```python
from build123d import *

# Parameters (mm, degrees)
SKETCH1_W           = 304.8
SKETCH1_H           = 50.8
BOSS_EXTRUDE1_DEPTH = 6.35
SKETCH2_W           = 41.275
SKETCH2_H           = 22.225
CUT_EXTRUDE1_DEPTH  = 265.034300402
SKETCH5_W           = 25.4
SKETCH5_H           = 6.35
BOSS_EXTRUDE2_DEPTH = 6.35
LPATTERN1_COUNT     = 6
LPATTERN1_PITCH     = 50.8
SKETCH6_W           = 6.35
SKETCH6_H           = 12.7
BOSS_EXTRUDE3_DEPTH = 6.35
LPATTERN2_COUNT     = 2
LPATTERN2_PITCH     = 38.1
CUT_EXTRUDE2_DEPTH  = 272.024068837
CUT_EXTRUDE3_DEPTH  = 272.024068837
SKETCH9_R           = 2.0955
CUT_EXTRUDE4_DEPTH  = 272.024068837


with BuildPart() as part:
    # Sketch1 → Boss-Extrude1 (new body)
    with BuildSketch(Plane.XY):
        with Locations((-110.333, 0)):
            Rectangle(SKETCH1_W, SKETCH1_H)
    extrude(amount=BOSS_EXTRUDE1_DEPTH)

    # Sketch2 → Cut-Extrude1 (cut, through all)
    with BuildSketch(Plane.XY.offset(6.35)):
        Rectangle(SKETCH2_W, SKETCH2_H)
    extrude(amount=-CUT_EXTRUDE1_DEPTH, mode=Mode.SUBTRACT)

    # Sketch5 → Boss-Extrude2 (add)
    with BuildSketch(Plane.XZ.offset(25.4)):
        with Locations((3.967, 3.175)):
            Rectangle(SKETCH5_W, SKETCH5_H)
    boss_extrude2 = extrude(amount=BOSS_EXTRUDE2_DEPTH)

    # LPattern1: Boss-Extrude2 ×6
    with Locations(*[(-i * LPATTERN1_PITCH, 0, 0) for i in range(1, LPATTERN1_COUNT)]):
        add(boss_extrude2)

    # Sketch6 → Boss-Extrude3 (add)
    with BuildSketch(Plane.ZY.offset(262.733)):
        with Locations((3.175, 19.05)):
            Rectangle(SKETCH6_W, SKETCH6_H)
    boss_extrude3 = extrude(amount=BOSS_EXTRUDE3_DEPTH)

    # LPattern2: Boss-Extrude3 ×2
    with Locations(*[(0, -i * LPATTERN2_PITCH, 0) for i in range(1, LPATTERN2_COUNT)]):
        add(boss_extrude3)

    # Sketch7 → Cut-Extrude2 (cut, through all)
    with BuildSketch(Plane.XY.offset(6.35)):
        Polygon((-262.733, 2.1336), (-262.733, -2.1336), (-253.97, -2.1336), (-253.97, -4.445), (-250.795, -4.445), (-250.795, -2.1336), (-247.493, -2.1336), (-247.493, 2.1336), (-250.795, 2.1336), (-250.795, 4.445), (-253.97, 4.445), (-253.97, 2.1336), align=None)
    extrude(amount=-CUT_EXTRUDE2_DEPTH, mode=Mode.SUBTRACT)

    # Sketch8 → Cut-Extrude3 (cut, through all)
    with BuildSketch(Plane.XY.offset(6.35)):
        Polygon((-226.7666, -25.4), (-222.4994, -25.4), (-222.4994, -16.637), (-220.188, -16.637), (-220.188, -13.462), (-222.4994, -13.462), (-222.4994, -10.16), (-226.7666, -10.16), (-226.7666, -13.462), (-229.078, -13.462), (-229.078, -16.637), (-226.7666, -16.637), align=None)
        Polygon((-125.1666, -25.4), (-120.8994, -25.4), (-120.8994, -16.637), (-118.588, -16.637), (-118.588, -13.462), (-120.8994, -13.462), (-120.8994, -10.16), (-125.1666, -10.16), (-125.1666, -13.462), (-127.478, -13.462), (-127.478, -16.637), (-125.1666, -16.637), align=None)
        Polygon((27.2334, -25.4), (31.5006, -25.4), (31.5006, -16.637), (33.812, -16.637), (33.812, -13.462), (31.5006, -13.462), (31.5006, -10.16), (27.2334, -10.16), (27.2334, -13.462), (24.922, -13.462), (24.922, -16.637), (27.2334, -16.637), align=None)
    extrude(amount=-CUT_EXTRUDE3_DEPTH, mode=Mode.SUBTRACT)

    # Sketch9 → Cut-Extrude4 (cut, through all)
    with BuildSketch(Plane(origin=(0, 0, 0), x_dir=(-1, 0, 0), z_dir=(0, 0, -1))):
        with Locations((46.904309807, -28.575)):
            Circle(SKETCH9_R)
        with Locations((199.304309807, -28.575)):
            Circle(SKETCH9_R)
    extrude(amount=-CUT_EXTRUDE4_DEPTH, mode=Mode.SUBTRACT)


solid = part.part
```
CAD build for the part. Positions are in the model's coordinates, mm. A direction names the side the tool comes from. Round coordinates to 2 decimals unless told otherwise and drop trailing zeros. Order: outer loops, then holes, each group sorted by start corner. A loop starts at its lowest first (then second) coordinate and runs counter-clockwise, first axis right, second up. Notation, with made-up numbers: (33, -36.75) - (53, -36.75) arc R26 ccw to (53, -15.75) - close; hole circle Ø9 at (62, 3.5). An arc over 180 degrees is marked (long way). Answer as CSV lines item,"result". Start each with the question number.
1. Saw through at A-A, the plane y = -20. Write the cut outline in (x, z).
2. Pin check, flat tips, straight feed: pin 1 (1.2 mm diameter, centred on x = 32.5, z = 4.5, fed in from -Y); pin 2 (1.8 mm diameter, centred on y = 3.5, z = 2, fed in from -X). Stop position of each tip, or through.
3. Drill centre lines: L1, parallel to X at y = -26, z = 4.75; L2, parallel to X at y = -11, z = 6; L3, parallel to X at y = -4, z = 1 (1 decimal). Where is each one in solid material? Low to high. Write a range as [from, to].
4. Pull direction X, two halves, no side cores. Call faces 6 (the face through (-161.133, -29, 3)), 7 (the face through (16.667, -29, 3)), 8 (the face through (37, -25.4, 3)): +X half, -X half, draft (parallel to the pull), parting line (faces both ways), or undercut.
5. Saw through at C-C, the plane y = -7. Write the cut outline in (x, z).
6. Saw through at B-B, the plane x = -6. Write the cut outline in (y, z), and give its area (3 significant figures).
7. Tool access for faces 1 (the face through (-262.733, 7, 3)), 2 (the face through (-237.333, -29, 3)), 3 (the face through (-20.638, 0, 3)), 4 (the face through (-266, -25.4, 3)), 5 (the face through (-111, -4, 6.35)): list every direction of +Z, -Z, +X, -X, +Y, -Y with a clear straight run to the whole face (end or side of a thin tool).
8. Saw through at D-D, the plane z = 2.75. Count the separate pieces of the cut face and the enclosed holes in it, and give its area (3 significant figures).
Model answer:
1,outline,"(-269.08, 0) - (-226.77, 0) - (-226.77, 6.35) - (-269.08, 6.35) - close; (-222.5, 0) - (-125.17, 0) - (-125.17, 6.35) - (-222.5, 6.35) - close; (-120.9, 0) - (27.23, 0) - (27.23, 6.35) - (-120.9, 6.35) - close; (31.5, 0) - (42.07, 0) - (42.07, 6.35) - (31.5, 6.35) - close"
2,pin 1,"stops at y = -25.4"
2,pin 2,"stops at x = -262.73"
3,L1,"x = [-262.73, -237.33], [-211.93, -186.53], [-161.13, -135.73], [-110.33, -84.93], [-59.53, -34.13], [-8.73, 16.67]"
3,L2,"x = [-262.73, -226.77], [-222.5, -125.17], [-120.9, -20.64], [20.64, 27.23], [31.5, 42.07]"
3,L3,"x = [-262.7, -254], [-250.8, -20.6], [20.6, 42.1]"
4,face 6,"undercut"
4,face 7,"+X half"
4,face 8,"draft"
5,outline,"(-262.73, 0) - (-20.64, 0) - (-20.64, 6.35) - (-262.73, 6.35) - close; (20.64, 0) - (42.07, 0) - (42.07, 6.35) - (20.64, 6.35) - close"
6,outline,"(-31.75, 0) - (-11.11, 0) - (-11.11, 6.35) - (-31.75, 6.35) - close; (11.11, 0) - (25.4, 0) - (25.4, 6.35) - (11.11, 6.35) - close"
6,area,"222 mm²"
7,face 1,"+Z, -Z, -X"
7,face 2,"+Z, -Z, -Y"
7,face 3,"+Z, -Z"
7,face 4,"+Z, -Z, -X, -Y"
7,face 5,"+Z, +X, -X, +Y, -Y"
8,separate pieces,"1"
8,enclosed holes,"3"
8,area,"15,300 mm²"
